from build123d import *

# Parameters (mm, degrees)
SKETCH_R           = 3.5
PAD_DEPTH          = 4
SKETCH001_W        = 4
SKETCH001_H        = 3
PAD001_DEPTH       = 15
POLARPATTERN_COUNT = 4
PAD002_DEPTH       = 15
PAD004_DEPTH       = 4
PAD005_DEPTH       = 20


with BuildPart() as part:
    # Sketch → Pad (new body)
    with BuildSketch(Plane.XY):
        Polygon((-9.8, 2), (-9.8, -2), (-2, -9.8), (2, -9.8), (9.8, -2), (9.8, 2), (2, 9.8), (-2, 9.8), align=None)
        Circle(SKETCH_R, mode=Mode.SUBTRACT)
    extrude(amount=-PAD_DEPTH)

    # Sketch001 → Pad001 (join)
    with BuildSketch(Plane.XY):
        with Locations((0, 8.3)):
            Rectangle(SKETCH001_W, SKETCH001_H)
    pad001 = extrude(amount=PAD001_DEPTH)

    # PolarPattern: Pad001 ×4 about axis
    polarpattern_axis = Axis((0, 0, 0), (0, 0, 1))
    for i in range(1, POLARPATTERN_COUNT):
        add(pad001.rotate(polarpattern_axis, i * 360 / POLARPATTERN_COUNT))

    # Sketch002 → Pad002 (join)
    with BuildSketch(Plane.XY):
        Polygon((-2, 9.8), (-5, 49.8), (5, 49.8), (2, 9.8), align=None)
    extrude(amount=PAD002_DEPTH)

    # Sketch002 → Pad004 (join)
    with BuildSketch(Plane.XY):
        Polygon((-2, 9.8), (-5, 49.8), (5, 49.8), (2, 9.8), align=None)
    extrude(amount=-PAD004_DEPTH)

    # Sketch003 → Pad005 (join, symmetric)
    with BuildSketch(Plane.YZ):
        Polygon((46.449787, 15), (91.155095, 15), (91.155095, 11), (51.155095, 11), (55.56327, -14), (51.56327, -14), align=None)
    extrude(amount=PAD005_DEPTH, both=True)


solid = part.part
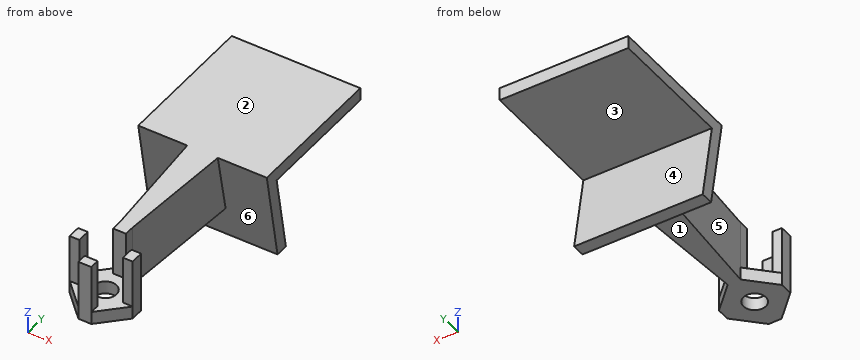
Can you work these out from the model? Positions are in its coordinate system, mm. Face numbers are marked on the shaded views. A direction names the side the tool comes from. Give positions to 0.01 mm unless a question says otherwise; leave off trailing zeros. Loops run counter-clockwise (first coordinate to the right, second up) from the corner with the lowest first, then second, coordinate; pieces in that order, holes last. Notation, with made-up numbers: M 57,-26.5 L 116,-26.5 A30 cw 116,5.5 Z; hole C 10,77 d2. An arc over 180 degrees is marked long. One line per item, written item: value. Start each with the question number.
1) If we section it at B-B, the plane y = 0: Write out the boundary of the cut face in (x, z).
2) On a 3-axis mill with a long thin cutter (end or side, diameter ignored), from which of +Z, -Z, +X, -X, +Y, -Y can I reach the whole of each face in a straight line? I mean the marked faces 1 and 2. Say none if no direction works.
3) If we section it at C-C, the plane z = 5: Write out the boundary of the cut face in (x, y), and give its area (3 significant figures).
4) If I drill on line 1 (Z direction, x = 3.5, y = 1); line 2 (Z direction, x = -7.5, y = 68.5); line 3 (X direction, y = 8, z = 13.75), over which ranges is the centre line in solid material (lowest first)? Write a range as [from, to].
5) I'm going to push flat-ended pins straight in: pin 1 (1.2 mm diameter, centred on x = 0.5, z = 7.5, fed in from +Y); pin 2 (5 mm diameter, centred on x = 11.5, z = -10.5, fed in from +Y); pin 3 (3 mm diameter, centred on y = 0.5, z = 2, fed in from +X); pin 4 (1 mm diameter, centred on x = -6, y = 31, fed in from +Z). Where does each tip first touch, or does it pass through?
6) Thinking about a two-plate mould opening in Y: for the marked faces 3, 4, 5 and 6, which applies, +Y half, -Y half, draft (parallel to the pull), parting line (faces both ways), or undercut?
7) If we section it at D-D, the plane x = -13: Write out the boundary of the cut face in (y, z).
8) If we section it at A-A, the plane x = 0: Write out the boundary of the cut face in (y, z).
Completed:
1. outline: M -9.8,-4 L -3.5,-4 L -3.5,0 L -6.8,0 L -6.8,15 L -9.8,15 Z; M 3.5,-4 L 9.8,-4 L 9.8,15 L 6.8,15 L 6.8,0 L 3.5,0 Z
2. face 1: -Z, +X, -X, -Y
2. face 2: +Z, +X, -X, +Y, -Y
3. outline: M -20,48.21 L -4.88,48.21 L -2,9.8 L -2,6.8 L 2,6.8 L 2,9.8 L 4.88,48.21 L 20,48.21 L 20,52.21 L -20,52.21 Z; M -9.8,-2 L -6.8,-2 L -6.8,2 L -9.8,2 Z; M -2,-9.8 L 2,-9.8 L 2,-6.8 L -2,-6.8 Z; M 6.8,-2 L 9.8,-2 L 9.8,2 L 6.8,2 Z
3. area: 472 mm^2
4. line 1: z = [-4, 0]
4. line 2: z = [11, 15]
4. line 3: x = [-2, 2]
5. pin 1: stops at y = 51.88
5. pin 2: stops at y = 55.39
5. pin 3: stops at x = 9.8
5. pin 4: passes through
6. face 3: draft
6. face 4: +Y half
6. face 5: undercut
6. face 6: undercut
7. outline: M 46.45,15 L 51.56,-14 L 55.56,-14 L 51.16,11 L 91.16,11 L 91.16,15 Z
8. outline: M -9.8,-4 L -3.5,-4 L -3.5,0 L -6.8,0 L -6.8,15 L -9.8,15 Z; M 3.5,-4 L 49.8,-4 L 51.56,-14 L 55.56,-14 L 51.16,11 L 91.16,11 L 91.16,15 L 6.8,15 L 6.8,0 L 3.5,0 Z
